Read the model definition and answer for the solid it produces. Units are mm, in the model's axes. Coordinates: 2 decimals unless noted, no trailing zeros. Loops run counter-clockwise (first coordinate to the right, second up) from the corner with the lowest first, then second, coordinate; pieces in that order, holes last. Notation, with made-up numbers: (40.5, -12) - (75.5, -12) arc R31 ccw to (75.5, 19) - close; hole circle Ø7 at (-16.5, 19.25). An arc over 180 degrees is marked (long way). One line per question, with ' | ' between items. Start each with the question number.
```python
from build123d import *

# Parameters (mm, degrees)
F0_R     = 17.375
F1_DEPTH = 3
F2_R     = 4.5
F3_DEPTH = 25.4
F4_R     = 1.406737
F5_DEPTH = 25


with BuildPart() as f1:
    # F0 (on Top) → F1 (new body)
    with BuildSketch(Plane.XY):
        Circle(F0_R)
    extrude(amount=F1_DEPTH)

    # F2 (on face) → F3 (cut)
    with BuildSketch(Plane.XY.offset(3)):
        Circle(F2_R)
    extrude(amount=-F3_DEPTH, mode=Mode.SUBTRACT)

    # F4 (on Top) → F5 (cut)
    with BuildSketch(Plane.XY):
        with Locations((-7.30325, 10.177708)):
            Circle(F4_R)
    extrude(amount=F5_DEPTH, mode=Mode.SUBTRACT)


solid = f1.part
```
1) The part is cut by section C-C on z = 1.05. Write down the section's boundary in (x, y) (3 decimals), and give its area (3 significant figures).
2) The mould has two halves that part along Y. Classify faces 1 (the cylindrical face through (-7.49, 11.57, 1.48)), 2 (the flat face through (4, -4, 0)), 3 (the cylindrical face through (9.34, 14.65, 1.48)): released by +Y, released by -Y, zero draft, split by the parting line, or undercut.
3) Given pin 1 Ø1.5 at (y, z) = (-13.5, 2.5) entering from +X, flat-ended and moving along its own axis, determine where the tip first touches the part or whether it passes through.
4) The part is cut by section D-D on x = 13. Write down the section's boundary in (y, z), and give its area (3 significant figures).
5) The part is cut by section A-A on x = 0. Write down the section's boundary in (y, z) (3 decimals).
6) Find the intervals of material crossed by line 1 along Y through (x, z) = (0, 1.25) (3 decimals); line 2 along X through (y, z) = (10, 0.3); line 3 along X through (y, z) = (1.5, 0.3), in increasing order. Write a range as from..to.
Answer below:
1) outline: circle Ø34.75 at (0, 0); hole circle Ø2.813 at (-7.303, 10.178); hole circle Ø9 at (0, 0) | area: 879 mm2
2) face 1: undercut | face 2: zero draft | face 3: split by the parting line
3) pin 1: x = 11.8
4) outline: (-11.53, 0) - (11.53, 0) - (11.53, 3) - (-11.53, 3) - close | area: 69.2 mm2
5) outline: (-17.375, 0) - (-4.5, 0) - (-4.5, 3) - (-17.375, 3) - close; (4.5, 0) - (17.375, 0) - (17.375, 3) - (4.5, 3) - close
6) line 1: -17.375..-4.5, 4.5..17.375 | line 2: -14.21..-8.7, -5.91..14.21 | line 3: -17.31..-4.24, 4.24..17.31
